from build123d import *

# Parameters (mm, degrees)
SKETCH2_W              = 9
SKETCH2_H              = 30
BOSS_EXTRUDE1_DEPTH    = 3
M5X0_8_TAPPED_HOLE1_D  = 4.2
SKETCH6_W              = 3
SKETCH6_H              = 30
BOSS_EXTRUDE2_DEPTH    = 18
CONVERT_SOLID5_START   = -30
CONVERT_SOLID5_DEPTH   = 30
CONVERT_SOLID5_2_DEPTH = 30
SKETCH24_W             = 3
SKETCH24_H             = 12
BOSS_EXTRUDE3_DEPTH    = 10
SKETCH21_R             = 2.5
CUT_EXTRUDE1_DEPTH     = 3


# Read off the part's stored shape, not the designer's step: Convert-Solid5
with BuildPart() as part:
    # Sketch2 → Boss-Extrude1 (new body)
    with BuildSketch(Plane(origin=(0, 0, 0), x_dir=(1, 0, 0), z_dir=(0, 1, 0))):
        with Locations((4.5, 15)):
            Rectangle(SKETCH2_W, SKETCH2_H)
    extrude(amount=BOSS_EXTRUDE1_DEPTH)

    # M5x0.8 Tapped Hole1 (through all)
    with Locations(Plane(origin=(0, 3, 0), x_dir=(1, 0, 0), z_dir=(0, 1, 0))):
        with Locations((6, 25), (6, 5)):
            Hole(M5X0_8_TAPPED_HOLE1_D / 2)

    # Sketch6 → Boss-Extrude2 (add)
    with BuildSketch(Plane(origin=(0, 0, 0), x_dir=(1, 0, 0), z_dir=(0, 1, 0))):
        with Locations((-1.5, 15)):
            Rectangle(SKETCH6_W, SKETCH6_H)
    extrude(amount=BOSS_EXTRUDE2_DEPTH)

    # Convert-Solid5 outline → Convert-Solid5 (cut)
    with BuildSketch(Plane.XY.offset(CONVERT_SOLID5_START)):
        with BuildLine():
            Line((-3, 0), (3, 0))
            ThreePointArc((3, 0), (-1.242640687, 1.757359313), (-3, 6))
            Line((-3, 6), (-3, 0))
        make_face()
    extrude(amount=CONVERT_SOLID5_DEPTH, mode=Mode.SUBTRACT)

    # Convert-Solid5 2 outline → Convert-Solid5 2 (add)
    with BuildSketch(Plane.XY.offset(CONVERT_SOLID5_START)):
        with BuildLine():
            Line((0, 3), (3, 3))
            ThreePointArc((3, 3), (0.878679656, 3.878679656), (0, 6))
            Line((0, 6), (0, 3))
        make_face()
    extrude(amount=CONVERT_SOLID5_2_DEPTH)

    # Sketch24 → Boss-Extrude3 (add)
    with BuildSketch(Plane.XY):
        with Locations((-1.5, 12)):
            Rectangle(SKETCH24_W, SKETCH24_H)
    extrude(amount=BOSS_EXTRUDE3_DEPTH)

    # Sketch21 → Cut-Extrude1 (cut)
    with BuildSketch(Plane(origin=(0, 0, 0), x_dir=(0, 0, -1), z_dir=(1, 0, 0))):
        with Locations((-5, 11.5)):
            Circle(SKETCH21_R)
        with Locations((15, 11.5)):
            Circle(SKETCH21_R)
    extrude(amount=-CUT_EXTRUDE1_DEPTH, mode=Mode.SUBTRACT)


solid = part.part
The listing builds one solid part. Answer for the finished solid, in the listing's coordinates (mm). A direction names the side the tool comes from. Give positions to 0.01 mm unless a question says otherwise; leave off trailing zeros. Loops run counter-clockwise (first coordinate to the right, second up) from the corner with the lowest first, then second, coordinate; pieces in that order, holes last. Notation, with made-up numbers: (-15, -27.5) - (34, -27.5) arc R25 ccw to (34, -5.5) - close; hole circle Ø1 at (3.5, 49.5). An arc over 180 degrees is marked (long way). Write each question's results on one line, items separated by ' | '.
1. Which of the six approach directions +Z, -Z, +X, -X, +Y, -Y give full straight-line access (tool end or side, diameter ignored) to faces 1 (the face through (3, 2, 0)), 2 (the face through (6, 3, -15)), 3 (the face through (-2, 18, -10))?
Resolved:
face 1: +Z, +X, -X, -Y | face 2: +Z, -Z, +X, +Y | face 3: +Z, -Z, +X, -X, +Y
2. Find section A-A, the plane y = 11.5. Write down the section's boundary in (x, z), then the cut area to 3 significant figures.
Resolved:
outline: (-3, -30) - (0, -30) - (0, -17.5) - (-3, -17.5) - close; (-3, -12.5) - (0, -12.5) - (0, 2.5) - (-3, 2.5) - close; (-3, 7.5) - (0, 7.5) - (0, 10) - (-3, 10) - close | area: 90.0 mm^2
3. For a pull along X with two mould halves and no side action, classify faces 4 (the face through (0.9, 3.86, -15.21)), 5 (the face through (-1, 10, -13)), 6 (the face through (4.87, 1.48, -26.77)) as +X half, -X half, draft (parallel to the pull), parting line (faces both ways), or undercut.
Resolved:
face 4: +X half | face 5: draft | face 6: undercut
4. Flat-ended cylindrical pins translate along their axes: P1, Ø6.5, axis at x = 7, z = -14, coming from the +Y side; P2, Ø3.5, axis at x = 6, z = -25, coming from the +Y side; P3, Ø3.5, axis at y = 10, z = -5, coming from the +X side; P4, Ø1.5, axis at x = -1, z = 7, coming from the -Y side. Find the tip coordinate at first contact, or state that the pin passes through.
Resolved:
P1: stops at y = 3 | P2: passes through | P3: stops at x = 0 | P4: stops at y = 6
5. Find section B-B, the plane x = 6. Write down the section's boundary in (y, z).
Resolved:
outline: (0, -30) - (3, -30) - (3, -27.1) - (0, -27.1) - close; (0, -22.9) - (3, -22.9) - (3, -7.1) - (0, -7.1) - close; (0, -2.9) - (3, -2.9) - (3, 0) - (0, 0) - close
6. Find section C-C, the plane z = 5. Write down the section's boundary in (x, y), then the cut area to 3 significant figures.
Resolved:
outline: (-3, 6) - (0, 6) - (0, 9) - (-3, 9) - close; (-3, 14) - (0, 14) - (0, 18) - (-3, 18) - close | area: 21.0 mm^2
7. Find section D-D, the plane z = -2. Write down the section's boundary in (x, y), then the cut area to 3 significant figures.
Resolved:
outline: (-3, 6) arc R6 ccw to (3, 0) - (9, 0) - (9, 3) - (3, 3) arc R3 cw to (0, 6) - (0, 18) - (-3, 18) - close | area: 75.2 mm^2
8. Consider probe 1 along Z at (x, y) = (6, 2); probe 2 along X at (y, z) = (13.75, -9.5); probe 3 along X at (y, z) = (2.35, -25). Determine where each line is inside the solid, lowest interval first. Write a range as from..to.
Resolved:
probe 1: z = -30..-27.1, -22.9..-7.1, -2.9..0 | probe 2: x = -3..0 | probe 3: x = -1.76..3.9, 8.1..9
